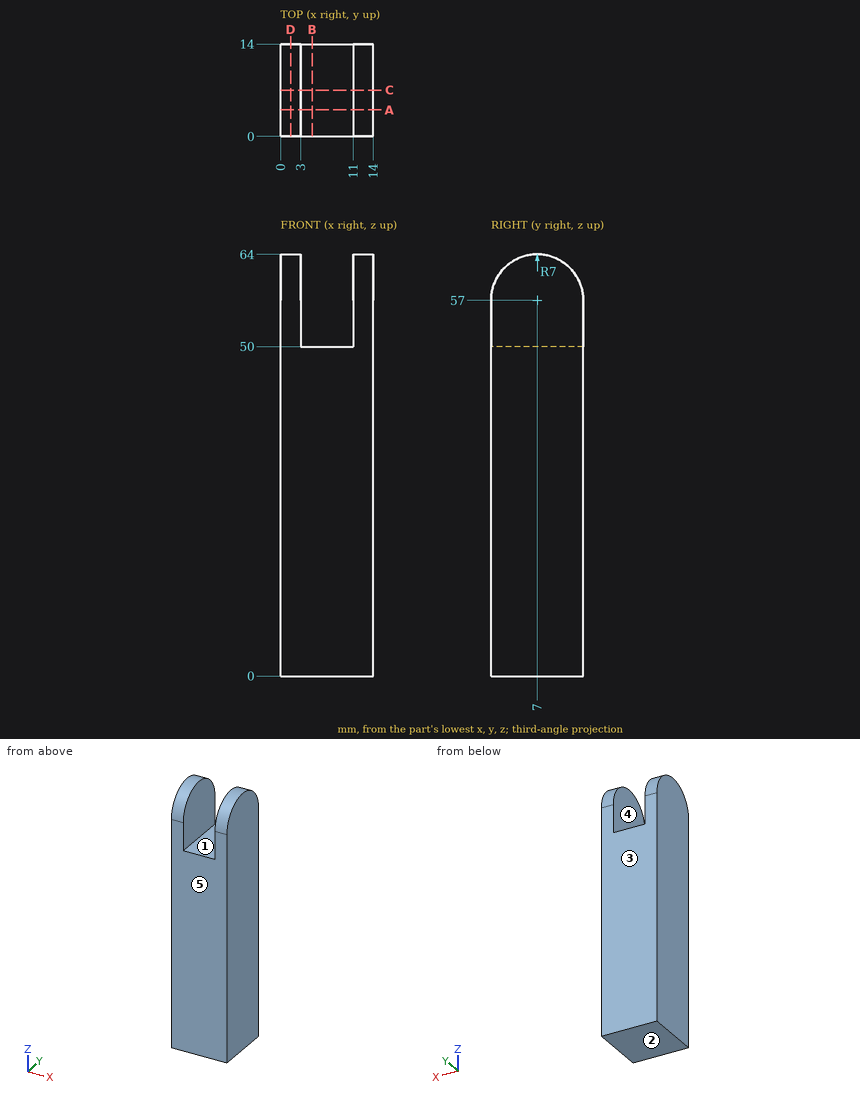
Verification items for this drawing (mm, ordinates from the low corner). A direction names the side the tool comes from. Coordinates: 2 decimals unless noted, no trailing zeros. Write each loop counter-clockwise with the first axis right and the second up, starting at its lowest first coordinate (ties: lowest second). Pieces come first, ordered by that corner, then holes. Notation, with made-up numbers: M 84,28 L 141,28 A15 ccw 141,35 Z; hole C 42,-27 d11. An arc over 180 degrees is marked long. Use CSV: the item, a comma, the result in double quotes.
Q1. Thickness scan on line 1 along X through (y, z) = (9.25, 55.5); line 2 along Z through (x, y) = (6.25, 5.25); line 3 along Z through (x, y) = (12, 6.75). Record the ranges inside material, lowest first. Write a range as [from, to].
Computed values:
line 1,"[0, 3], [11, 14]"
line 2,"[0, 50]"
line 3,"[0, 64]"
Q2. Section check A-A, the plane y = 4. Enter the section's corners in (x, z).
Computed values:
outline,"M 0,0 L 14,0 L 14,63.32 L 11,63.32 L 11,50 L 3,50 L 3,63.32 L 0,63.32 Z"
Q3. Mould release check, pull along Z, two halves, no side actions. Record for the marked faces 1, 2 and 3: pulls with the +Z half, pulls with the -Z half, needs draft (parallel to the pull), parting line crosses it, or undercut.
Computed values:
face 1,"pulls with the +Z half"
face 2,"pulls with the -Z half"
face 3,"needs draft"
Q4. Go/stop test with a flat-tipped pin: P1, Ø4, axis at x = 7, y = 9, coming from the +Z side. Record where the tip stops, or that it passes through.
Computed values:
P1,"z = 50"
Q5. Set-up check for the marked faces 4 and 5: record each of +Z, -Z, +X, -X, +Y, -Y from which the full face is reachable in a straight line by a thin tool's end or side.
Computed values:
face 4,"+Z, +Y, -Y"
face 5,"+Z, -Z, +X, -X, -Y"
Q6. Section check D-D, the plane x = 1.5. Enter the section's corners in (y, z).
Computed values:
outline,"M 0,0 L 14,0 L 14,57 A7 ccw 0,57 Z"
Q7. Section check C-C, the plane y = 7. Enter the section's corners in (x, z).
Computed values:
outline,"M 0,0 L 14,0 L 14,64 L 11,64 L 11,50 L 3,50 L 3,64 L 0,64 Z"
Q8. Section check B-B, the plane x = 4.75. Enter the section's corners in (y, z).
Computed values:
outline,"M 0,0 L 14,0 L 14,50 L 0,50 Z"
